Here's how the part is built. I have some questions about the finished solid (model axes, mm). A direction names the side the tool comes from. Round coordinates to 2 decimals unless told otherwise and drop trailing zeros. Order: outer loops, then holes, each group sorted by start corner. A loop starts at its lowest first (then second) coordinate and runs counter-clockwise, first axis right, second up. Notation, with made-up numbers: (61, -11.5) -> (81, -11.5) arc R17 cw to (81, 9.5) -> close; hole circle Ø6 at (71.25, 14.5). An arc over 180 degrees is marked (long way). Use a Markdown table: item, result. Add a question column.
from build123d import *

# Parameters (mm, degrees)
F0_R     = 1.6
F0_R_2   = 6.5
F1_DEPTH = 1.9
F2_R     = 1.6
F3_DEPTH = 1.2


# Not quite as in the source:
# - a feature names something its author has since deleted; it is built from what else it names


with BuildPart() as f1:
    # F0 (on Top) → F1 (new body)
    with BuildSketch(Plane.XY):
        with BuildLine():
            Line((15.7910159975, 25.3955767816), (11.1241112417, 30.0624815375))
            Line((11.1241112417, 30.0624815375), (2.7910159975, 30.0624815375))
            ThreePointArc((2.7910159975, 30.0624815375), (2.0839092163, 29.7695883186), (1.7910159975, 29.0624815375))
            Line((1.7910159975, 29.0624815375), (1.7910159975, 25.0624815375))
            Line((1.7910159975, 25.0624815375), (-20.2089840025, 25.0624815375))
            Line((-20.2089840025, 25.0624815375), (-20.2089840025, 29.0624815375))
            ThreePointArc((-20.2089840025, 29.0624815375), (-20.5018772213, 29.7695883186), (-21.2089840025, 30.0624815375))
            Line((-21.2089840025, 30.0624815375), (-29.5420792466, 30.0624815375))
            Line((-29.5420792466, 30.0624815375), (-34.2089840025, 25.3955767816))
            Line((-34.2089840025, 25.3955767816), (-34.2089840025, -15.2706137067))
            Line((-34.2089840025, -15.2706137067), (-29.5420792466, -19.9375184625))
            Line((-29.5420792466, -19.9375184625), (-21.2089840025, -19.9375184625))
            ThreePointArc((-21.2089840025, -19.9375184625), (-20.5018772213, -19.6446252437), (-20.2089840025, -18.9375184625))
            Line((-20.2089840025, -18.9375184625), (-20.2089840025, -14.9375184625))
            Line((-20.2089840025, -14.9375184625), (1.7910159975, -14.9375184625))
            Line((1.7910159975, -14.9375184625), (1.7910159975, -18.9375184625))
            ThreePointArc((1.7910159975, -18.9375184625), (2.0839092163, -19.6446252437), (2.7910159975, -19.9375184625))
            Line((2.7910159975, -19.9375184625), (11.1241112417, -19.9375184625))
            Line((11.1241112417, -19.9375184625), (15.7910159975, -15.2706137067))
            Line((15.7910159975, -15.2706137067), (15.7910159975, 25.3955767816))
        make_face()
        with Locations((-29.7089840025, -14.1875184625)):
            Circle(F0_R, mode=Mode.SUBTRACT)
        with Locations((-24.4589840025, -10.1875184625)):
            Circle(F0_R, mode=Mode.SUBTRACT)
        with Locations((11.2910159975, -14.1875184625)):
            Circle(F0_R, mode=Mode.SUBTRACT)
        with Locations((6.0410159975, -10.1875184625)):
            Circle(F0_R, mode=Mode.SUBTRACT)
        with Locations((-24.4589840025, 20.3124815375)):
            Circle(F0_R, mode=Mode.SUBTRACT)
        with Locations((-29.7089840025, 24.3124815375)):
            Circle(F0_R, mode=Mode.SUBTRACT)
        with Locations((-9.2089840025, 5.0624815375)):
            Circle(F0_R_2, mode=Mode.SUBTRACT)
        with Locations((6.0410159975, 20.3124815375)):
            Circle(F0_R, mode=Mode.SUBTRACT)
        with Locations((11.2910159975, 24.3124815375)):
            Circle(F0_R, mode=Mode.SUBTRACT)
    extrude(amount=F1_DEPTH)

    # F2 (on face) → F3 (cut)
    with BuildSketch(Plane.XY.offset(1.9)):
        Polygon((-30.6354453237, 27.7700822596), (-33.1665847246, 25.2389428587), (-32.2401234033, 21.7813421366), (-28.7825226812, 20.8548808153), (-26.2513832804, 23.3860202162), (-27.1778446016, 26.8436209383), align=None)
        with Locations((-29.7089840025, 24.3124815375)):
            Circle(F2_R, mode=Mode.SUBTRACT)
        Polygon((14.7486167196, 25.2389428587), (12.2174773188, 27.7700822596), (8.7598765967, 26.8436209383), (7.8334152754, 23.3860202162), (10.3645546763, 20.8548808153), (13.8221553984, 21.7813421366), align=None)
        with Locations((11.2910159975, 24.3124815375)):
            Circle(F2_R, mode=Mode.SUBTRACT)
        Polygon((12.2174773188, -17.6451191847), (14.7486167196, -15.1139797838), (13.8221553984, -11.6563790617), (10.3645546763, -10.7299177404), (7.8334152754, -13.2610571413), (8.7598765967, -16.7186578634), align=None)
        with Locations((11.2910159975, -14.1875184625)):
            Circle(F2_R, mode=Mode.SUBTRACT)
        Polygon((-33.1665847246, -15.1139797838), (-30.6354453237, -17.6451191847), (-27.1778446016, -16.7186578634), (-26.2513832804, -13.2610571413), (-28.7825226812, -10.7299177404), (-32.2401234033, -11.6563790617), align=None)
        with Locations((-29.7089840025, -14.1875184625)):
            Circle(F2_R, mode=Mode.SUBTRACT)
    extrude(amount=-F3_DEPTH, mode=Mode.SUBTRACT)


solid = f1.part
(1) I want a section at A-A on y = 10. List the corners of the cut face in (x, z) for me, and give its area (3 significant figures).
(2) Please list where these lines run through material, in increasing order: probe 1 along X at (y, z) = (-10.5, 1.5); probe 2 along X at (y, z) = (-9.5, 0.5); probe 3 along Y at (x, z) = (12.5, 0.4). Write a range as from..to.
(3) On a 3-axis mill with a long thin cutter (end or side, diameter ignored), from which of +Z, -Z, +X, -X, +Y, -Y can I reach the whole of each face in a straight line? I mean faces 5 (the flat face through (-15, 11, 0)), 6 (the flat face through (1.791, -17, 1)), 7 (the flat face through (-28.88, 27.3, 1.31)). Say none if no direction works.
(4) I want a section at B-B on x = -17. List the corners of the cut face in (y, z) for me.
(5) I'm going to push flat-ended pins straight in: P1, Ø0.6, axis at x = -9.5, z = 1, coming from the -Y side; P2, Ø0.6, axis at y = -17, z = 1, coming from the +X side; P3, Ø1, axis at x = -8.5, z = 1.5, coming from the +Y side. Where does each tip first touch, or does it pass through?
(6) I want a section at C-C on z = 1.55. State how many separate pieces and enclosed holes the cut face has, and give its area (3 significant figures).
(7) If we mould it in two halves opening along Y, with no side actions, what happens to faces 1 (the flat face through (-30.536, 21.325, 1.308)), 2 (the flat face through (12.12, -11.2, 1.31)), 3 (the flat face through (-9, -14.938, 1)), 4 (the flat face through (1.791, 27, 1))? For each: pulls with the +Y half, pulls with the -Y half, needs draft (parallel to the pull), parting line crosses it, or undercut.
Output:
| question | item | result |
|---|---|---|
| 1 | outline | (-34.21, 0) -> (-13.44, 0) -> (-13.44, 1.9) -> (-34.21, 1.9) -> close; (-4.98, 0) -> (15.79, 0) -> (15.79, 1.9) -> (-4.98, 1.9) -> close |
| 1 | area | 78.9 mm² |
| 2 | probe 1 | -34.21..-26.03, -22.89..4.47, 7.61..15.79 |
| 2 | probe 2 | -34.21..-25.9, -23.01..4.6, 7.49..15.79 |
| 2 | probe 3 | -18.56..-15.24, -13.14..23.26, 25.36..28.69 |
| 3 | face 5 | -Z, +X, -X, +Y, -Y |
| 3 | face 6 | +Z, -Z, -Y |
| 3 | face 7 | +Z |
| 4 | outline | (-14.94, 0) -> (25.06, 0) -> (25.06, 1.9) -> (-14.94, 1.9) -> close |
| 5 | P1 | y = -14.94 |
| 5 | P2 | x = 14.36 |
| 5 | P3 | y = 25.06 |
| 6 | separate pieces | 1 |
| 6 | enclosed holes | 9 |
| 6 | area | 1,940 mm² |
| 7 | face 1 | undercut |
| 7 | face 2 | undercut |
| 7 | face 3 | pulls with the -Y half |
| 7 | face 4 | needs draft |
